from build123d import *

# Parameters (mm, degrees)
F2_DEPTH = 3


with BuildPart() as f2:
    # F1 (on Front) → F2 (new body)
    with BuildSketch(Plane.XZ):
        Polygon((-33.941125497, 6.058874503), (-40, 0), (40, 0), (33.941125497, 6.058874503), (29.6984848098, 10.3015151902), (0, 40), (-29.6984848098, 10.3015151902), align=None)
        Polygon((29.6984848098, 10.3015151902), (33.941125497, 6.058874503), (36.0624458405, 8.1801948466), (31.8198051534, 12.4228355337), align=None)
        Polygon((-36.0624458405, 8.1801948466), (-33.941125497, 6.058874503), (-29.6984848098, 10.3015151902), (-31.8198051534, 12.4228355337), align=None)
    extrude(amount=F2_DEPTH)


solid = f2.part
Input: part model. Units: mm. Frame: model coordinates. A direction names the side the tool comes from. Give positions to 0.01 mm unless a question says otherwise; leave off trailing zeros. Order: outer loops, then holes, each group sorted by start corner. A loop starts at its lowest first (then second) coordinate and runs counter-clockwise, first axis right, second up.
Q1. Set-up query: faces 1 (the flat face through (37, -1, 3)), 2 (the flat face through (-33.91, -1.48, 10.33)), 3 (the flat face through (-35.017, -1.479, 7.134)), 4 (the flat face through (30.774, -1.479, 11.377)). Return all of +Z, -Z, +X, -X, +Y, -Y with unobstructed straight access to the full face (end or side cutting, diameter ignored); none if empty.
Checked values:
face 1: +X, +Y, -Y
face 2: +Z, -X, +Y, -Y
face 3: -X, +Y, -Y
face 4: +Z, +Y, -Y
Q2. Ray query, probe 1 along X at (y, z) = (-0.15, 12); probe 2 along Z at (x, y) = (12.5, -2.7); probe 3 along X at (y, z) = (-2.65, 29.5). Return the intervals inside material, ascending.
Checked values:
probe 1: x = -32.24 to -31.4, -28 to 28, 31.4 to 32.24
probe 2: z = 0 to 27.5
probe 3: x = -10.5 to 10.5
Q3. Section D-D on z = 18. Output: boundary loops of the cut face in (x, y), and give its area (3 significant figures).
Checked values:
outline: (-22, -3) - (22, -3) - (22, 0) - (-22, 0) - close
area: 132 mm2
Q4. Section B-B on z = 11.5. Output: boundary loops of the cut face in (x, y), and give its area (3 significant figures).
Checked values:
outline: (-32.74, -3) - (-30.9, -3) - (-30.9, 0) - (-32.74, 0) - close; (-28.5, -3) - (28.5, -3) - (28.5, 0) - (-28.5, 0) - close; (30.9, -3) - (32.74, -3) - (32.74, 0) - (30.9, 0) - close
area: 182 mm2
Q5. Section A-A on y = -1.25. Output: boundary loops of the cut face in (x, z), and give its area (3 significant figures).
Checked values:
outline: (-40, 0) - (40, 0) - (33.94, 6.06) - (36.06, 8.18) - (31.82, 12.42) - (29.7, 10.3) - (0, 40) - (-29.7, 10.3) - (-31.82, 12.42) - (-36.06, 8.18) - (-33.94, 6.06) - close
area: 1,640 mm2
Q6. Contact query for flat-ended pins moving along their axis: pin 1 Ø1.5 at (y, z) = (-0.5, 24) entering from -X; pin 2 Ø1 at (y, z) = (-1.5, 31.5) entering from -X; pin 3 Ø1 at (x, y) = (22, -1.5) entering from +Z. Output: stop coordinate, or through.
Checked values:
pin 1: stops at x = -16.75
pin 2: stops at x = -9
pin 3: stops at z = 18.5
Q7. Section C-C on x = -14. Output: boundary loops of the cut face in (y, z), and give its area (3 significant figures).
Checked values:
outline: (-3, 0) - (0, 0) - (0, 26) - (-3, 26) - close
area: 78.0 mm2
